For this review, use the dimensioned drawing (mm, ordinates from the lowest corner) and the shaded views. A direction names the side the tool comes from. Coordinates: 2 decimals unless noted, no trailing zeros. Loops run counter-clockwise (first coordinate to the right, second up) from the corner with the lowest first, then second, coordinate; pieces in that order, holes last. Notation, with made-up numbers: M -37,-20.75 L -27,-20.75 A7 ccw -27,-15.75 Z; hole C 4,-26.75 d6. An arc over 180 degrees is marked long. One line per item, written item: value.
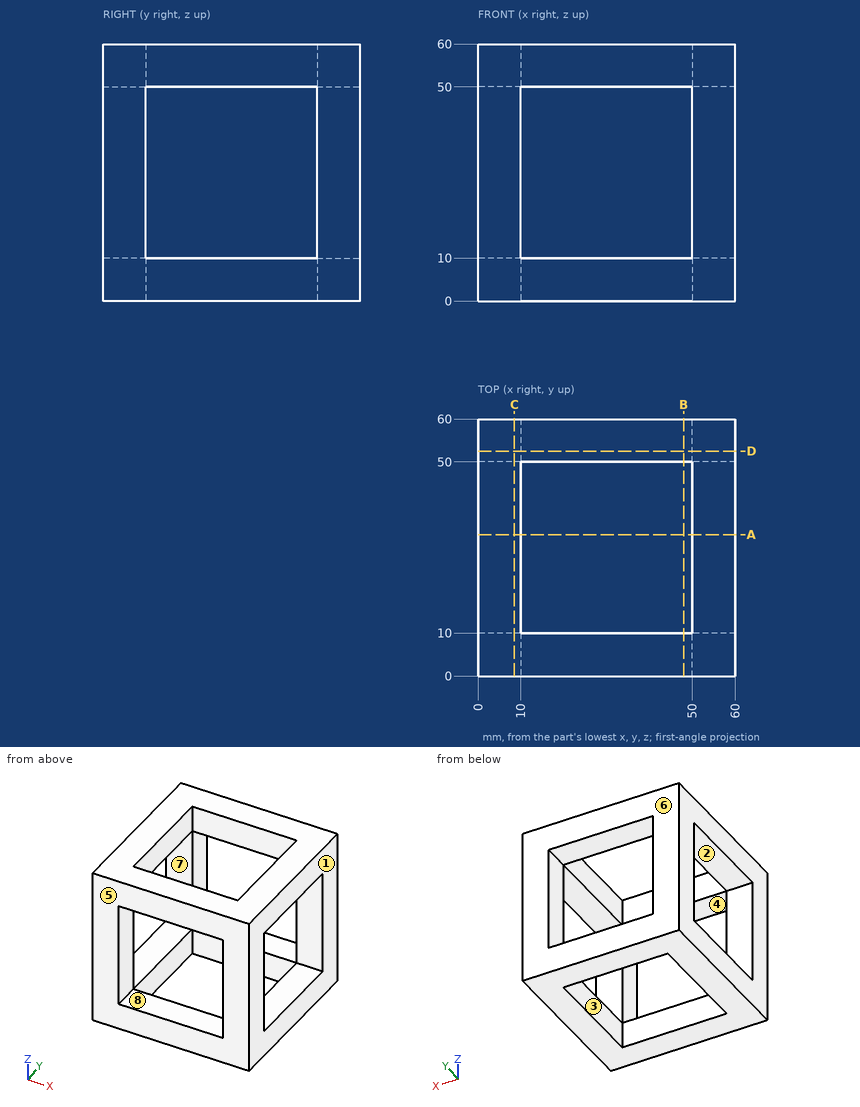
(1) Insertion check: pin 1 Ø5 at (x, z) = (29.5, 14) entering from +Y. The pin has a flat end and moves straight along its axis. Give the tip position at first contact, or say it passes through.
Checks:
pin 1: through
(2) Tool access review of the marked faces 1, 2, 3 and 4: name each direction out of +Z, -Z, +X, -X, +Y, -Y from which nothing blocks a thin tool from reaching the whole face with its end or side.
Checks:
face 1: +Z, -Z, +X, +Y, -Y
face 2: +X, -X
face 3: +Z, -Z
face 4: +Y, -Y
(3) Add section A-A on y = 33. State the section outline as (x, z) points, then the cut area to 3 significant figures.
Checks:
outline: M 0,0 L 10,0 L 10,10 L 0,10 Z; M 0,50 L 10,50 L 10,60 L 0,60 Z; M 50,0 L 60,0 L 60,10 L 50,10 Z; M 50,50 L 60,50 L 60,60 L 50,60 Z
area: 400 mm^2
(4) Add section C-C on x = 8.5. State the section outline as (y, z) points.
Checks:
outline: M 0,0 L 60,0 L 60,60 L 0,60 Z; hole M 10,10 L 50,10 L 50,50 L 10,50 Z
(5) Draft analysis for pull direction Y (two halves, no side actions). For the marked faces 5, 6, 7 and 8, state which applies: pulls with the +Y half, pulls with the -Y half, needs draft (parallel to the pull), parting line crosses it, or undercut.
Checks:
face 5: pulls with the -Y half
face 6: pulls with the +Y half
face 7: undercut
face 8: needs draft
(6) To check wall thickness, follow L1, parallel to Y at x = 54, z = 14.5. State the ranges of the line that lie inside material, in increasing order. Write a range as [from, to].
Checks:
L1: [0, 10], [50, 60]
